from build123d import *

# Parameters (mm, degrees)
SKETCH2_R                                 = 71.4375
BOSS_EXTRUDE1_DEPTH                       = 188.4934
BOSS_EXTRUDE4_START                       = -188.4934
SKETCH2_3_R                               = 6.35
BOSS_EXTRUDE4_DEPTH                       = 59.1566
BOSS_EXTRUDE2_START                       = -76.2
BOSS_EXTRUDE2_DEPTH                       = 2.54
SKETCH5_W                                 = 4.365625
SKETCH5_H                                 = 147.6375
F_11_32_0_34375_DIAMETER_HOLE1_AT_2_COUNT = 2
F_11_32_0_34375_DIAMETER_HOLE1_AT_2_PITCH = 69.85
F_11_32_0_34375_DIAMETER_HOLE1_AT_3_COUNT = 2
F_11_32_0_34375_DIAMETER_HOLE1_AT_3_PITCH = 128.577700244
F_11_32_0_34375_DIAMETER_HOLE1_AT_4_COUNT = 2
F_11_32_0_34375_DIAMETER_HOLE1_AT_4_PITCH = 107.95
BOSS_EXTRUDE3_START                       = 71.0438
BOSS_EXTRUDE3_DEPTH                       = 142.0876
CUT_EXTRUDE1_START                        = -119.937949444
CUT_EXTRUDE1_DEPTH                        = 55.725898888
BOSS_EXTRUDE5_START                       = -188.4934
SKETCH8_R                                 = 2.413
BOSS_EXTRUDE5_DEPTH                       = 31.75


# Read off the part's stored shape, not the designer's step: Cut-Extrude1
with BuildPart() as part:
    # Sketch2 → Boss-Extrude1 (new body)
    with BuildSketch(Plane.XY):
        Circle(SKETCH2_R)
    extrude(amount=-BOSS_EXTRUDE1_DEPTH)

    # Sketch2<3> → Boss-Extrude4 (add)
    with BuildSketch(Plane.XY.offset(BOSS_EXTRUDE4_START)):
        Circle(SKETCH2_3_R)
    extrude(amount=-BOSS_EXTRUDE4_DEPTH)



with BuildPart() as body_2:
    # Sketch3 → Boss-Extrude2 (new body)
    with BuildSketch(Plane(origin=(0, 0, 0), x_dir=(1, 0, 0), z_dir=(0, 1, 0)).offset(BOSS_EXTRUDE2_START)):
        with BuildLine():
            Line((-53.975, 144.0688), (53.975, 144.0688))
            ThreePointArc((53.975, 144.0688), (66.044464227, 139.069464227), (71.0438, 127))
            Line((71.0438, 127), (71.0438, 57.15))
            ThreePointArc((71.0438, 57.15), (66.044464227, 45.080535773), (53.975, 40.0812))
            Line((53.975, 40.0812), (-53.975, 40.0812))
            ThreePointArc((-53.975, 40.0812), (-66.044464227, 45.080535773), (-71.0438, 57.15))
            Line((-71.0438, 57.15), (-71.0438, 127))
            ThreePointArc((-71.0438, 127), (-66.044464227, 139.069464227), (-53.975, 144.0688))
        make_face()
    extrude(amount=BOSS_EXTRUDE2_DEPTH)

    # Sketch5 → 11/32 (0.34375) Diameter Hole1 (revolve, cut)
    with BuildSketch(Plane(origin=(-53.975, -76.2, -127), x_dir=(0, 0, -1), z_dir=(1, 0, 0))):
        with Locations((2.1828125, 73.81875)):
            Rectangle(SKETCH5_W, SKETCH5_H)
    f_11_32_0_34375_diameter_hole1 = revolve(axis=Axis((-53.975, -82.55, -127), (0, 1, 0)), mode=Mode.SUBTRACT)

    # 11/32 (0.34375) Diameter Hole1 at 2: 11/32 (0.34375) Diameter Hole1 ×2
    with Locations(*[(0, 0, i * F_11_32_0_34375_DIAMETER_HOLE1_AT_2_PITCH) for i in range(1, F_11_32_0_34375_DIAMETER_HOLE1_AT_2_COUNT)]):
        add(f_11_32_0_34375_diameter_hole1, mode=Mode.SUBTRACT)

    # 11/32 (0.34375) Diameter Hole1 at 3: 11/32 (0.34375) Diameter Hole1 ×2
    with Locations(*[Vector(0.8395701571521513, 0, 0.543251278157274) * (i * F_11_32_0_34375_DIAMETER_HOLE1_AT_3_PITCH) for i in range(1, F_11_32_0_34375_DIAMETER_HOLE1_AT_3_COUNT)]):
        add(f_11_32_0_34375_diameter_hole1, mode=Mode.SUBTRACT)

    # 11/32 (0.34375) Diameter Hole1 at 4: 11/32 (0.34375) Diameter Hole1 ×2
    with Locations(*[(i * F_11_32_0_34375_DIAMETER_HOLE1_AT_4_PITCH, 0, 0) for i in range(1, F_11_32_0_34375_DIAMETER_HOLE1_AT_4_COUNT)]):
        add(f_11_32_0_34375_diameter_hole1, mode=Mode.SUBTRACT)


with BuildPart() as part_1:
    add(part.part)

    add(body_2.part)  # Boss-Extrude3 merges body 2
    # Sketch6 → Boss-Extrude3 (add)
    with BuildSketch(Plane(origin=(0, 0, 0), x_dir=(0, 0, -1), z_dir=(1, 0, 0)).offset(BOSS_EXTRUDE3_START)):
        Polygon((64.212050556, -73.66), (74.6125, -45.085), (109.5375, -45.085), (119.937949444, -73.66), align=None)
    extrude(amount=-BOSS_EXTRUDE3_DEPTH)

    # Cut-Extrude1 outline → Cut-Extrude1 (cut)
    with BuildSketch(Plane.XY.offset(CUT_EXTRUDE1_START)):
        Polygon((-71.0438, -73.66), (-55.413528865, -45.085), (-71.0438, -45.085), align=None)
    cut_extrude1 = extrude(amount=CUT_EXTRUDE1_DEPTH, mode=Mode.SUBTRACT)

    # Mirror2: Cut-Extrude1 across plane
    add(cut_extrude1.mirror(Plane(origin=(0, 0, 0), x_dir=(0, 0, 1), z_dir=(1, 0, 0))), mode=Mode.SUBTRACT)

    # Sketch8 → Boss-Extrude5 (add)
    with BuildSketch(Plane.XY.offset(BOSS_EXTRUDE5_START)):
        with Locations((46.0375, -46.0375)):
            Circle(SKETCH8_R)
        with Locations((46.0375, 46.0375)):
            Circle(SKETCH8_R)
        with Locations((-46.0375, 46.0375)):
            Circle(SKETCH8_R)
        with Locations((-46.0375, -46.0375)):
            Circle(SKETCH8_R)
    extrude(amount=-BOSS_EXTRUDE5_DEPTH)


solid = part_1.part
Work out the finished part from the listing and answer in its coordinate system (mm). A direction names the side the tool comes from. Give positions to 0.01 mm unless a question says otherwise; leave off trailing zeros. Order: outer loops, then holes, each group sorted by start corner. A loop starts at its lowest first (then second) coordinate and runs counter-clockwise, first axis right, second up. Notation, with made-up numbers: (70.25, -30.5) -> (107.25, -30.5) arc R19 ccw to (107.25, 4.5) -> close; hole circle Ø4 at (4, -3.75). An arc over 180 degrees is marked (long way). One line per item, written item: value.
Item 1: Find section B-B, the plane z = -97. Give the vertices of the cut face in (x, y) (1 decimal), plus the area to 3 significant figures.
Answer sheet:
outline: (-71, -76.2) -> (71, -76.2) -> (71, -73.7) -> (55.4, -45.1) arc R71.4 ccw (long way) to (-55.4, -45.1) -> (-71, -73.7) -> close
area: 18,000 mm²
Item 2: Flat-ended cylindrical pins translate along their axes: P1, Ø3, axis at x = -20, y = -75.5, coming from the -Z side; P2, Ø2, axis at x = 0.5, y = -74.5, coming from the +Z side; P3, Ø2.5, axis at x = -46.5, y = 46, coming from the -Z side; P4, Ø1, axis at x = -8, z = -199.5, coming from the -Y side. Find the tip coordinate at first contact, or state that the pin passes through.
Answer sheet:
P1: z = -144.07
P2: z = -40.08
P3: z = -220.24
P4: through
Item 3: Find section C-C, the plane x = -25.5. Give the vertices of the cut face in (y, z), plus the area to 3 significant figures.
Answer sheet:
outline: (-76.2, -144.07) -> (-73.66, -144.07) -> (-73.66, -119.94) -> (-66.73, -117.42) -> (-66.73, -188.49) -> (66.73, -188.49) -> (66.73, 0) -> (-66.73, 0) -> (-66.73, -66.73) -> (-73.66, -64.21) -> (-73.66, -40.08) -> (-76.2, -40.08) -> close
area: 25,800 mm²
Item 4: Determine the mould class of faces 5 (the flat face through (1, -76.2, -93)), 6 (the flat face through (63.338, -59.573, -92.465)), 7 (the cylindrical face through (-65.91, -74.95, -44.95)) for opening direction Y: released by +Y, released by -Y, zero draft, split by the parting line, or undercut.
Answer sheet:
face 5: released by -Y
face 6: undercut
face 7: zero draft
Item 5: Straight lines are drawn through the part: probe 1 along X at (y, z) = (-74.6, -57.15); probe 2 along Z at (x, y) = (42, 33); probe 3 along Y at (x, z) = (17, -50). For each, find the intervals that lie inside material, in ascending order.
Answer sheet:
probe 1: -71.04 to -58.34, -49.61 to 49.61, 58.34 to 71.04
probe 2: -188.49 to 0
probe 3: -76.2 to -73.66, -69.39 to 69.39
Item 6: Find section A-A, the plane y = 0. Give the vertices of the cut face in (x, z).
Answer sheet:
outline: (-71.44, -188.49) -> (-6.35, -188.49) -> (-6.35, -247.65) -> (6.35, -247.65) -> (6.35, -188.49) -> (71.44, -188.49) -> (71.44, 0) -> (-71.44, 0) -> close
Item 7: Find section D-D, the plane x = 0. Give the vertices of the cut face in (y, z).
Answer sheet:
outline: (-76.2, -144.07) -> (-73.66, -144.07) -> (-73.66, -119.94) -> (-71.44, -119.13) -> (-71.44, -188.49) -> (-6.35, -188.49) -> (-6.35, -247.65) -> (6.35, -247.65) -> (6.35, -188.49) -> (71.44, -188.49) -> (71.44, 0) -> (-71.44, 0) -> (-71.44, -65.02) -> (-73.66, -64.21) -> (-73.66, -40.08) -> (-76.2, -40.08) -> close
Item 8: A tool of negligible diameter and unlimited length cuts with its end or side. For faces 1 (the cylindrical face through (-1.38, -6.2, -217.66)), 2 (the cylindrical face through (53.78, -74.91, -52.79)), 3 (the cylindrical face through (65.91, -74.95, -139.2)), 4 (the cylindrical face through (-66.176, -74.948, -138.936)), from which of +Z, -Z, +X, -X, +Y, -Y can it reach the whole face along a straight path? Write none if from no direction.
Answer sheet:
face 1: -Z
face 2: -Y
face 3: -Z, +X, -Y
face 4: -Z, -X, -Y
